```python
from build123d import *

# Parameters (mm, degrees)
SKETCH152_R     = 1.7
PAD084_DEPTH    = 3
CHAMFER055_SIZE = 1
SKETCH154_R     = 1.6
SKETCH154_W     = 15
SKETCH154_H     = 17
POCKET_DEPTH    = 215.688564
CHAMFER057_SIZE = 1
SKETCH178_R     = 1.6
POCKET024_DEPTH = 3.001


with BuildPart() as part:
    # Sketch152 → Pad084 (new body)
    with BuildSketch(Plane.XY):
        Polygon((40, -30), (-40, -30), (-40, 30), (-30, 30), (-30, 40), (30, 40), (30, 30), (40, 30), align=None)
        with Locations((0, 35)):
            Circle(SKETCH152_R, mode=Mode.SUBTRACT)
        with Locations((-35, 0)):
            Circle(SKETCH152_R, mode=Mode.SUBTRACT)
        with Locations((35, 0)):
            Circle(SKETCH152_R, mode=Mode.SUBTRACT)
    extrude(amount=PAD084_DEPTH)

    # Chamfer055
    chamfer055_edges = [part.edges().sort_by_distance(p)[0] for p in [
        (40, 30, 1.5),
        (30, 40, 1.5),
        (-30, 40, 1.5),
        (-40, 30, 1.5),
        (-40, -30, 1.5),
        (40, -30, 1.5),
    ]]
    chamfer(chamfer055_edges, length=CHAMFER055_SIZE)


with BuildPart() as part_1:
    # Body072 placement: moved
    add(part.part.moved(Location((0, 34.999969, 320.000031))))

    # Sketch154 (on Face5 of Clone) → Pocket (cut, through all)
    with BuildSketch(Plane(origin=(0, 34.999969, 323.000031), x_dir=(1, 0, 0), z_dir=(0, 0, 1))):
        with Locations((-21.5, -26)):
            Circle(SKETCH154_R)
        with Locations((-21.5, 4)):
            Circle(SKETCH154_R)
        with Locations((-21.5, -11)):
            Rectangle(SKETCH154_W, SKETCH154_H)
    pocket = extrude(amount=-POCKET_DEPTH, mode=Mode.SUBTRACT)

    # Mirrored: Pocket across Sketch154 V_Axis
    add(pocket.mirror(Plane(origin=(0, 34.999969, 323.000031), x_dir=(0, 0, 1), z_dir=(1, 0, 0))), mode=Mode.SUBTRACT)

    # Chamfer057
    chamfer057_edges = [part_1.edges().sort_by_distance(p)[0] for p in [
        (29, 15.499969, 321.500031),
        (29, 32.499969, 321.500031),
        (14, 32.499969, 321.500031),
        (14, 15.499969, 321.500031),
        (-14, 15.499969, 321.500031),
        (-29, 15.499969, 321.500031),
        (-29, 32.499969, 321.500031),
        (-14, 32.499969, 321.500031),
    ]]
    chamfer(chamfer057_edges, length=CHAMFER057_SIZE)

    # Sketch178 (on Face39 of Chamfer057) → Pocket024 (cut, through all)
    with BuildSketch(Plane(origin=(0, 34.999969, 323.000031), x_dir=(1, 0, 0), z_dir=(0, 0, 1))):
        with Locations((-25, 21.16)):
            Circle(SKETCH178_R)
        with Locations((25, 21.16)):
            Circle(SKETCH178_R)
        with Locations((15, 21.16)):
            Circle(SKETCH178_R)
        with Locations((1, 21.16)):
            Circle(SKETCH178_R)
        with BuildLine():
            ThreePointArc((-18.491423, 27.506442), (-19.905637, 26.920655), (-20.491423, 25.506442))
            Line((-20.491423, 16.813558), (-20.491423, 25.506442))
            ThreePointArc((-20.491423, 16.813558), (-19.905637, 15.399345), (-18.491423, 14.813558))
            Line((-8.105475, 14.813558), (-18.491423, 14.813558))
            ThreePointArc((-8.105475, 14.813558), (-6.691261, 15.399345), (-6.105475, 16.813558))
            Line((-6.105475, 25.506442), (-6.105475, 16.813558))
            ThreePointArc((-6.105475, 25.506442), (-6.691261, 26.920655), (-8.105475, 27.506442))
            Line((-18.491423, 27.506442), (-8.105475, 27.506442))
        make_face()
    extrude(amount=-POCKET024_DEPTH, mode=Mode.SUBTRACT)


solid = part_1.part
```
Part model, mm, in its own coordinate system. A direction names the side the tool comes from. Round coordinates to 2 decimals unless told otherwise and drop trailing zeros. Write each loop counter-clockwise with the first axis right and the second up, starting at its lowest first coordinate (ties: lowest second). Pieces come first, ordered by that corner, then holes. Notation, with made-up numbers: M 14,27.25 L 71,27.25 A19 cw 71,54.25 Z; hole C 72.25,22.25 d7. An arc over 180 degrees is marked long. Answer as CSV lines item,"result". Start each with the question number.
1) Which spindle directions (+Z, -Z, +X, -X, +Y, -Y) get a long thin tool onto all of the face, cutting with end or side? Do faces 1 (the face through (-20.491, 56, 322)), 2 (the face through (1, 40, 323)). Say none if no direction does.
2) Band-saw the part on A-A (y = 29.5). List the corners of the cut face in (x, z).
3) Drill centre lines: L1, parallel to Y at x = 21.5, z = 321.45; L2, parallel to X at y = 29.5, z = 321.1; L3, parallel to Y at x = -25, z = 322.1. Where is each one in solid material? Low to high.
4) Band-saw the part on B-B (x = -25). List the corners of the cut face in (y, z), then the cut area to 3 significant figures.
5) Band-saw the part on D-D (x = 21.5). List the corners of the cut face in (y, z), then the cut area to 3 significant figures.
6) Mould opens along Y. For faces 3 (the face through (30, 70, 321)), 4 (the face through (1, 5, 321)), 5 (the face through (-29, 24, 322)) say: +Y half, -Y half, draft (parallel to the pull), parting line (faces both ways), or undercut.
7) Drop flat-ended pins along their axis: pin 1 (0.9 mm diameter, centred on x = 34, z = 321.5, fed in from +Y); pin 2 (0.9 mm diameter, centred on y = 70.5, z = 322, fed in from -X). Give the stop position or say it passes through.
8) Band-saw the part on C-C (x = -13). List the corners of the cut face in (y, z).
Worked out:
1,face 1,"+Z, -Z"
1,face 2,"+Z, +X, -X, +Y, -Y"
2,outline,"M -40,320 L -29,320 L -29,323 L -40,323 Z; M -14,320 L 14,320 L 14,323 L -14,323 Z; M 29,320 L 40,320 L 40,323 L 29,323 Z"
3,L1,"5 to 7.4, 10.6 to 15.5, 32.5 to 37.4, 40.6 to 75"
3,L2,"-40 to -29, -14 to 14, 29 to 40"
3,L3,"5 to 15.5, 32.5 to 54.56, 57.76 to 75"
4,outline,"M 5,320 L 15.5,320 L 15.5,323 L 5,323 Z; M 32.5,320 L 54.56,320 L 54.56,323 L 32.5,323 Z; M 57.76,320 L 75,320 L 75,323 L 57.76,323 Z"
4,area,"149 mm²"
5,outline,"M 5,320 L 7.4,320 L 7.4,323 L 5,323 Z; M 10.6,320 L 15.5,320 L 15.5,323 L 10.6,323 Z; M 32.5,320 L 37.4,320 L 37.4,323 L 32.5,323 Z; M 40.6,320 L 75,320 L 75,323 L 40.6,323 Z"
5,area,"140 mm²"
6,face 3,"draft"
6,face 4,"-Y half"
6,face 5,"undercut"
7,pin 1,"y = 65"
7,pin 2,"x = -30"
8,outline,"M 5,320 L 49.81,320 L 49.81,323 L 5,323 Z; M 62.51,320 L 75,320 L 75,323 L 62.51,323 Z"
